```python
from build123d import *

# Parameters (mm, degrees)
PAD_DEPTH    = 1.5
CHAMFER_SIZE = 1


with BuildPart() as part:
    # Sketch → Pad (new body)
    with BuildSketch(Plane.XY):
        with BuildLine():
            ThreePointArc((1.772002, 6.772002), (-4.949747, -4.949747), (6.772002, 1.772002))
            Line((6.772002, 1.772002), (9.491066, 4.491066))
            ThreePointArc((4.491066, 9.491066), (-7.424621, -7.424621), (9.491066, 4.491066))
            Line((1.772002, 6.772002), (4.491066, 9.491066))
        make_face()
    extrude(amount=PAD_DEPTH)

    # Chamfer
    chamfer_edges = [part.edges().sort_by_distance(p)[0] for p in [
        (-7.424621, -7.424621, 1.5),
    ]]
    chamfer(chamfer_edges, length=CHAMFER_SIZE)


solid = part.part
```
Model file for the job. Use its own axes, mm. A direction names the side the tool comes from. Round coordinates to 2 decimals unless told otherwise and drop trailing zeros. Order: outer loops, then holes, each group sorted by start corner. A loop starts at its lowest first (then second) coordinate and runs counter-clockwise, first axis right, second up. Notation, with made-up numbers: (-10.5, -19) -> (-1.5, -19) arc R22 ccw to (-1.5, 3) -> close; hole circle Ø6 at (37, 36.5). An arc over 180 degrees is marked (long way). Use one line per item in the form item = value.
Item 1: Cut at A-A, the plane y = 0. Write the cut outline in (x, z).
Returned:
outline = (-10.5, 0) -> (-7, 0) -> (-7, 1.5) -> (-9.5, 1.5) -> (-10.5, 0.5) -> close; (7, 0) -> (10.5, 0) -> (10.5, 0.5) -> (9.5, 1.5) -> (7, 1.5) -> close
Item 2: Flat gauge pin, fed straight in: pin 1 Ø5 at (x, y) = (-8, 6.5) entering from +Z. Where does the tip first touch, or does it go through?
Returned:
pin_1 = 1.5
Item 3: Tool access for faces 1 (the face through (-7.09, -6.56, 1.34)), 2 (the face through (8, 3, 1)): list every direction of +Z, -Z, +X, -X, +Y, -Y with a clear straight run to the whole face (end or side of a thin tool).
Returned:
face_1 = +Z
face_2 = +Z, -Z, +Y
Item 4: Cut at C-C, the plane z = 1.2. Write the cut outline in (x, y), and give its area (3 significant figures).
Returned:
outline = (1.77, 6.77) -> (3.96, 8.96) arc R9.8 ccw (long way) to (8.96, 3.96) -> (6.77, 1.77) arc R7 cw (long way) to start
area = 127 mm^2
Item 5: Drill centre lines: line 1 (X direction, y = 0, z = 0.45); line 2 (Y direction, x = 0, z = 0.85); line 3 (X direction, y = -4.75, z = 1.3). Where is each one in solid material? Low to high.
Returned:
line_1 = -10.5 to -7, 7 to 10.5
line_2 = -10.15 to -7, 7 to 10.15
line_3 = -8.46 to -5.14, 5.14 to 8.46
Item 6: Pull direction X, two halves, no side cores. Call faces 3 (the face through (-3.5, -6.3, 1.5)), 4 (the face through (3, 8, 1)), 5 (the face through (-5.127, -4.765, 0.74)): released by +X, released by -X, zero draft, split by the parting line, or undercut.
Returned:
face_3 = zero draft
face_4 = released by +X
face_5 = undercut
